Print and shaded views of the part. All mm, measured from the part's lowest x, y and z. A direction names the side the tool comes from. Coordinates: 2 decimals unless noted, no trailing zeros. Loops run counter-clockwise (first coordinate to the right, second up) from the corner with the lowest first, then second, coordinate; pieces in that order, holes last. Notation, with made-up numbers: M -36,-22 L -2,-22 A7 ccw -2,-10 Z; hole C 38.25,22.5 d4. An arc over 180 degrees is marked long. Use a Markdown table: item, result. Add a question column.
1) Band-saw the part on A-A (y = 24). List the corners of the cut face in (x, z), plus the area to 3 significant figures.
2) Band-saw the part on B-B (z = 7.5). List the corners of the cut face in (x, y).
3) Pin check, flat tips, straight feed: pin 1 Ø2 at (x, z) = (7, 9.5) entering from +Y; pin 2 Ø4.5 at (y, z) = (19.5, 5.5) entering from -X; pin 3 Ø6.5 at (x, z) = (19.5, 9) entering from -Y. Stop position of each tip, or through.
4) Pull direction X, two halves, no side cores. Call the marked faces 1, 2 and 3: released by +X, released by -X, zero draft, split by the parting line, or undercut.
5) Band-saw the part on D-D (x = 4). List the corners of the cut face in (y, z).
6) Wall check: probe 1 along X at (y, z) = (24, 12); probe 2 along Y at (x, z) = (23.5, 7.5); probe 3 along Y at (x, z) = (8.5, 5.5). Give the ranges that are in metal, low to high. Write a range as from..to.
7) Tool access for the marked faces 4, 5 and 6: list every direction of +Z, -Z, +X, -X, +Y, -Y with a clear straight run to the whole face (end or side of a thin tool).
8) Band-saw the part on C-C (y = 7.5). List the corners of the cut face in (x, z).
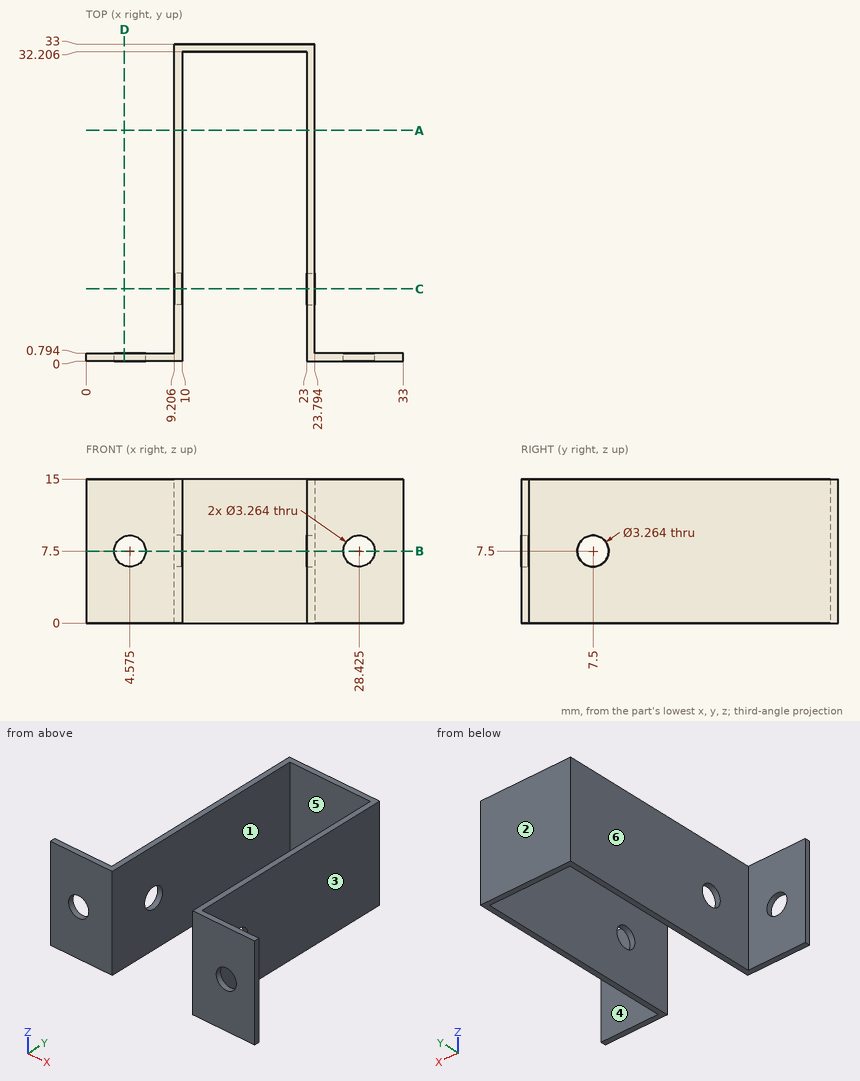
Entries:
| question | item | result |
|---|---|---|
| 1 | outline | M 9.21,0 L 10,0 L 10,15 L 9.21,15 Z; M 23,0 L 23.79,0 L 23.79,15 L 23,15 Z |
| 1 | area | 23.8 mm2 |
| 2 | outline | M 0,0 L 2.94,0 L 2.94,0.79 L 0,0.79 Z; M 6.21,0 L 10,0 L 10,5.87 L 9.21,5.87 L 9.21,0.79 L 6.21,0.79 Z; M 9.21,9.13 L 10,9.13 L 10,32.21 L 23,32.21 L 23,9.13 L 23.79,9.13 L 23.79,33 L 9.21,33 Z; M 23,0 L 26.79,0 L 26.79,0.79 L 23.79,0.79 L 23.79,5.87 L 23,5.87 Z; M 30.06,0 L 33,0 L 33,0.79 L 30.06,0.79 Z |
| 3 | pin 1 | y = 0.79 |
| 3 | pin 2 | x = 9.21 |
| 3 | pin 3 | y = 32.21 |
| 4 | face 1 | undercut |
| 4 | face 2 | zero draft |
| 4 | face 3 | released by +X |
| 5 | outline | M 0,0 L 0.79,0 L 0.79,5.97 L 0,5.97 Z; M 0,9.03 L 0.79,9.03 L 0.79,15 L 0,15 Z |
| 6 | probe 1 | 9.21..10, 23..23.79 |
| 6 | probe 2 | 0..5.87, 9.13..33 |
| 6 | probe 3 | 0..0.79 |
| 7 | face 4 | +Z, -Z, +X, +Y |
| 7 | face 5 | +Z, -Z, -Y |
| 7 | face 6 | +Z, -Z, -X, +Y |
| 8 | outline | M 9.21,0 L 10,0 L 10,5.87 L 9.21,5.87 Z; M 9.21,9.13 L 10,9.13 L 10,15 L 9.21,15 Z; M 23,0 L 23.79,0 L 23.79,5.87 L 23,5.87 Z; M 23,9.13 L 23.79,9.13 L 23.79,15 L 23,15 Z |
